Here's how the part is built. I have some questions about the finished solid (model axes, mm). A direction names the side the tool comes from. Coordinates: 2 decimals unless noted, no trailing zeros. Write each loop counter-clockwise with the first axis right and the second up, starting at its lowest first coordinate (ties: lowest second). Pieces come first, ordered by that corner, then holes.
Item 1: I'm going to push flat-ended pins straight in: pin 1 Ø8 at (x, z) = (-6.35, 14.3) entering from -Y; pin 2 Ø23 at (x, y) = (-31.75, 28.575) entering from -Z; pin 3 Ø8 at (x, z) = (-57.15, 14.3) entering from +Y (3 decimals). Where does each tip first touch, or does it pass through?
Item 2: If I drill on line 1 (Z direction, x = -21, y = 8) (3 decimals); line 2 (Z direction, x = -6.35, y = 1.55); line 3 (Y direction, x = -56.5, z = 22) (3 decimals), over which ranges is the centre line in solid material (lowest first)?
Item 3: If we section it at C-C (y = 22): Please give me the cut outline in (x, z) (3 decimals).
Item 4: If we section it at A-A (y = 9): Please give me the cut outline in (x, z) (3 decimals).
Item 5: If we section it at D-D (x = -31.75): Count the separate pieces of the cut face and the enclosed holes in it, then the cut area to 3 significant figures.
Item 6: For faces 1 (the face through (-32, 13, 3.175)), 2 (the face through (-5.858, 25.452, 90.535)), which set-ups out of +Z, -Z, +X, -X, +Y, -Y let a thin tool reach every point of the face, with its end or its side?
Item 7: We'd pull the mould along Y, two halves only. Please class faces 3 (the face through (-31, 13, 88.925)), 4 (the face through (-24.069, 40.622, 1.61)), 5 (the face through (-57.804, 25.1, 1.61)): +Y half, -Y half, draft (parallel to the pull), parting line (faces both ways), or undercut.
Item 8: If we section it at B-B (x = -21): Please give me the cut outline in (y, z) (3 decimals).
Autodesk Inventor part; units mm, degrees
ref_plane "YZ Plane" through (0, 0, 0) normal (1, 0, 0) x (0, 1, 0)
ref_plane "XZ Plane" through (0, 0, 0) normal (0, 1, 0) x (-1, 0, 0)
ref_plane "XY Plane" through (0, 0, 0) normal (0, 0, 1) x (1, 0, 0)
sketch "Sketch1" plane through (0, 0, 0) normal (0, 1, 0) x (-1, 0, 0)
  line L0 (0, 0) -> (63.5, 0)
  line L1 (63.5, 0) -> (63.5, 92.1004)
  line L2 (63.5, 92.1004) -> (0, 92.1004)
  line L3 (0, 92.1004) -> (0, 0)
  dimension "d0" = 92.1004
  dimension "d2" = 63.5
extrude "Plate1" add sketch "Sketch1" along normal blind 3.175
sketch "Sketch2" plane through (0, 0, 88.9254) normal (0, 0, 1) x (1, 0, 0)
  line L0 (-63.5, 0) -> (0, 0)
  line L1 (0, 0) -> (0, 50.8)
  line L2 (0, 50.8) -> (-63.5, 50.8)
  line L3 (-63.5, 50.8) -> (-63.5, 0)
edge flange "Flange1" height 50.8 angle 90 thickness 3.175 bend radius 3.175 thickness toward (0, 0, 1) relief tear relief width 3.175 relief depth 1.5875 corner gap 3.175 corner form 0 edges at (-31.75, 3.175, 92.1004) (-31.75, 3.175, 0) wall of the first edge with corners at (-63.5, 0, 88.9254) (0, 0, 88.9254) (0, 50.8, 88.9254) (-63.5, 50.8, 88.9254)
bend "Bend1"
corner "Corner1"
sketch "Sketch3" plane through (-63.5, 50.8, 92.1004) normal (0, 0, 1) x (1, 0, 0)
  line L0 (0, -44.45) -> (63.5, -44.45)
  line L1 (63.5, 0) -> (63.5, -44.45)
  line L2 (0, 0) -> (63.5, 0)
  line L3 (0, -44.45) -> (0, 0)
  circle A0 centre (31.75, -22.225) radius 14.2875
  arc A1 (51.9461, -12.9478) -> (11.5539, -12.9478) centre (31.75, -22.225) ccw
  line L4 (0, -38.1) -> (11.5539, -12.9478)
  line L5 (51.9461, -12.9478) -> (63.5, -38.1)
  point P0 (63.5, -50.8)
  dimension "d14" = 28.575
  dimension "d15" = 6.35
  dimension "d16" = 28.575
  dimension "d17" = 44.45
  dimension "d18" = 31.75
  dimension "d19" = 6.35
extrude "Cut1" cut sketch "Sketch3" against normal blind 2540 contours L3 L2 A1 L4 | L5 A1 L2 L1 | A0
sketch "Sketch4" plane through (0, 0, 0) normal (0, -1, 0) x (1, 0, 0)
  line L0 (0, 85.7504) -> (0, 6.35)
  line L1 (-63.5, 6.35) -> (-63.5, 85.7504)
  circle A0 centre (-57.15, 77.8002) radius 3.3782
  circle A1 centre (-6.35, 77.8002) radius 3.3782
  circle A2 centre (-57.15, 14.3002) radius 3.3782
  circle A3 centre (-6.35, 14.3002) radius 3.3782
  line L2 (-63.5, 46.0502) -> (0, 46.0502)
  point P0 (0, 0)
  dimension "d22" = 6.7564
  dimension "d23" = 6.7564
  dimension "d24" = 6.7564
  dimension "d25" = 6.7564
  dimension "d26" = 31.75
  dimension "d27" = 31.75
  dimension "d28" = 31.75
  dimension "d29" = 31.75
  dimension "d30" = 6.35
  dimension "d31" = 6.35
  dimension "d32" = 6.35
  dimension "d33" = 6.35
extrude "Cut2" cut sketch "Sketch4" against normal blind 3.175
equation "\"d34\" = Thickness"
equation "\"d4\" = BendReliefWidth"
equation "\"d5\" = BendReliefDepth"
equation "\"d6\" = MinimumRemnant"
equation "\"d7\" = BendRadius"
equation "\"d10\" = BendRadius"
equation "\"d11\" = CornerReliefSize"
equation "\"d12\" = GapSize"
equation "\"d13\" = JacobiRadiusSize"
equation "\"BendRadius\" = Thickness"
equation "\"BendReliefWidth\" = Thickness"
equation "\"BendReliefDepth\" = 0.5 * Thickness"
equation "\"CornerReliefSize\" = 4 * Thickness"
equation "\"MinimumRemnant\" = 2 * Thickness"
equation "\"TransitionRadius\" = BendRadius"
equation "\"JacobiRadiusSize\" = BendRadius"
equation "\"GapSize\" = Thickness"
equation "\"d3\" = BendRadius"
properties part number "Bearing Mount 5" material "Aluminum 6061"
Answer list:
1. pin 1: stops at y = 0
1. pin 2: passes through
1. pin 3: stops at y = 3.175
2. line 1: z = 0 to 3.175, 88.925 to 92.1
2. line 2: z = 2.19 to 10.92, 17.68 to 74.42, 81.18 to 89.91
2. line 3: y = 0 to 3.175
3. outline: (-59.228, 0) - (-44.435, 0) - (-44.435, 3.175) - (-59.228, 3.175) - close; (-59.228, 88.925) - (-44.435, 88.925) - (-44.435, 92.1) - (-59.228, 92.1) - close; (-19.065, 0) - (-4.272, 0) - (-4.272, 3.175) - (-19.065, 3.175) - close; (-19.065, 88.925) - (-4.272, 88.925) - (-4.272, 92.1) - (-19.065, 92.1) - close
4. outline: (-63.5, 0) - (0, 0) - (0, 3.175) - (-63.5, 3.175) - close; (-63.5, 88.925) - (0, 88.925) - (0, 92.1) - (-63.5, 92.1) - close
5. separate pieces: 3
5. enclosed holes: 0
5. area: 400 mm2
6. face 1: +X, -X, +Y
6. face 2: +Z, -Z, +X, +Y
7. face 3: draft
7. face 4: undercut
7. face 5: +Y half
8. outline: (0, 6.35) arc R6.35 ccw to (6.35, 0) - (19.164, 0) - (19.164, 3.175) - (6.35, 3.175) arc R3.175 cw to (3.175, 6.35) - (3.175, 85.75) arc R3.175 cw to (6.35, 88.925) - (19.164, 88.925) - (19.164, 92.1) - (6.35, 92.1) arc R6.35 ccw to (0, 85.75) - close; (37.986, 0) - (48.027, 0) - (48.027, 3.175) - (37.986, 3.175) - close; (37.986, 88.925) - (48.027, 88.925) - (48.027, 92.1) - (37.986, 92.1) - close
